Build history of the part. All positions in model axes, mm. A direction names the side the tool comes from. Coordinates: 2 decimals unless noted, no trailing zeros. Loops run counter-clockwise (first coordinate to the right, second up) from the corner with the lowest first, then second, coordinate; pieces in that order, holes last.
(1) Slice it at B-B (x = 5). Give the number of separate pieces and of enclosed holes in the cut face, and give its area (3 significant figures).
(2) Flat gauge pins, fed straight in: P1, Ø3, axis at x = 20.5, z = 56, coming from the +Y side; P2, Ø8, axis at x = 5.5, y = 6, coming from the +Z side; P3, Ø12, axis at x = 9.5, y = 16, coming from the +Z side. Where does each tip first touch, or does it go through?
(3) Slice it at C-C (z = 70). Give the cut face in (x, y).
(4) Tool access for faces 5 (the face through (25, -18, 32)), 6 (the face through (5, -45, 67)), 7 (the face through (3.7, 3.7, 3)): list every direction of +Z, -Z, +X, -X, +Y, -Y with a clear straight run to the whole face (end or side of a thin tool).
(5) Wall check: L1, parallel to X at y = 5, z = 16.25; L2, parallel to X at y = -47.6, z = 70; L3, parallel to Z at x = 20, y = -49.15. Give the ranges that are in metal, low to high.
(6) Slice it at A-A (y = 5). Give the cut face in (x, z), and give its area (3 significant figures).
(7) Two-plate mould, pull along Z, no slides. Class faces 1 (the face through (19, 18, 3)), 2 (the face through (19.792, -48.521, 71.586)), 3 (the face through (6.3, -47, 53.7)), 4 (the face through (12, 13, 0)): pulls with the +Z half, pulls with the -Z half, needs draft (parallel to the pull), parting line crosses it, or undercut.
from build123d import *

# Parameters (mm, degrees)
BOSS_EXTRUDE1_DEPTH = 25
CUT_EXTRUDE2_REACH  = 80
CUT_EXTRUDE2_START  = -3
SKETCH2_R           = 3
SKETCH2_R_2         = 1.6
CUT_EXTRUDE3_REACH  = 77
SKETCH2_3_R         = 1.6
CUT_EXTRUDE7_REACH  = 80
CUT_EXTRUDE7_START  = -3
SKETCH3_R           = 3
SKETCH3_R_2         = 1.6
CUT_EXTRUDE8_REACH  = 77
SKETCH3_3_R         = 1.6


with BuildPart() as part:
    # Sketch1 → Boss-Extrude1 (new body)
    with BuildSketch(Plane(origin=(0, 0, 0), x_dir=(0, 0, -1), z_dir=(1, 0, 0))):
        Polygon((0, 0), (-50, -50), (-75, -50), (0, 25), align=None)
    extrude(amount=BOSS_EXTRUDE1_DEPTH)

    # Sketch2 → Cut-Extrude2 (cut, up to next)
    with BuildSketch(Plane.XZ.offset(50).offset(CUT_EXTRUDE2_START), mode=Mode.PRIVATE) as cut_extrude2_sk1:
        with Locations((20, 70)):
            Circle(SKETCH2_R)
        with Locations((20, 70)):
            Circle(SKETCH2_R_2, mode=Mode.SUBTRACT)
    cut_extrude2_tool1 = extrude(cut_extrude2_sk1.sketch, amount=-CUT_EXTRUDE2_REACH, mode=Mode.PRIVATE) & part.part
    add(cut_extrude2_tool1.solids().sort_by_distance((17.084853, -47, 70))[0], mode=Mode.SUBTRACT)
    # Sketch2 → Cut-Extrude2 (cut, up to next)
    with BuildSketch(Plane.XZ.offset(50).offset(CUT_EXTRUDE2_START), mode=Mode.PRIVATE) as cut_extrude2_sk2:
        with Locations((5, 70)):
            Circle(SKETCH2_R)
        with Locations((5, 70)):
            Circle(SKETCH2_R_2, mode=Mode.SUBTRACT)
    cut_extrude2_tool2 = extrude(cut_extrude2_sk2.sketch, amount=-CUT_EXTRUDE2_REACH, mode=Mode.PRIVATE) & part.part
    add(cut_extrude2_tool2.solids().sort_by_distance((2.084853, -47, 70))[0], mode=Mode.SUBTRACT)
    # Sketch2 → Cut-Extrude2 (cut, up to next)
    with BuildSketch(Plane.XZ.offset(50).offset(CUT_EXTRUDE2_START), mode=Mode.PRIVATE) as cut_extrude2_sk3:
        with Locations((5, 55)):
            Circle(SKETCH2_R)
        with Locations((5, 55)):
            Circle(SKETCH2_R_2, mode=Mode.SUBTRACT)
    cut_extrude2_tool3 = extrude(cut_extrude2_sk3.sketch, amount=-CUT_EXTRUDE2_REACH, mode=Mode.PRIVATE) & part.part
    add(cut_extrude2_tool3.solids().sort_by_distance((2.084853, -47, 55))[0], mode=Mode.SUBTRACT)
    # Sketch2 → Cut-Extrude2 (cut, up to next)
    with BuildSketch(Plane.XZ.offset(50).offset(CUT_EXTRUDE2_START), mode=Mode.PRIVATE) as cut_extrude2_sk4:
        with Locations((20, 55)):
            Circle(SKETCH2_R)
        with Locations((20, 55)):
            Circle(SKETCH2_R_2, mode=Mode.SUBTRACT)
    cut_extrude2_tool4 = extrude(cut_extrude2_sk4.sketch, amount=-CUT_EXTRUDE2_REACH, mode=Mode.PRIVATE) & part.part
    add(cut_extrude2_tool4.solids().sort_by_distance((17.084853, -47, 55))[0], mode=Mode.SUBTRACT)

    # Sketch2_3 → Cut-Extrude3 (cut, up to next)
    with BuildSketch(Plane.XZ.offset(50), mode=Mode.PRIVATE) as cut_extrude3_sk1:
        with Locations((20, 70)):
            Circle(SKETCH2_3_R)
    cut_extrude3_tool1 = extrude(cut_extrude3_sk1.sketch, amount=-CUT_EXTRUDE3_REACH, mode=Mode.PRIVATE) & part.part
    add(cut_extrude3_tool1.solids().sort_by_distance((20, -50, 70))[0], mode=Mode.SUBTRACT)
    # Sketch2_3 → Cut-Extrude3 (cut, up to next)
    with BuildSketch(Plane.XZ.offset(50), mode=Mode.PRIVATE) as cut_extrude3_sk2:
        with Locations((5, 70)):
            Circle(SKETCH2_3_R)
    cut_extrude3_tool2 = extrude(cut_extrude3_sk2.sketch, amount=-CUT_EXTRUDE3_REACH, mode=Mode.PRIVATE) & part.part
    add(cut_extrude3_tool2.solids().sort_by_distance((5, -50, 70))[0], mode=Mode.SUBTRACT)
    # Sketch2_3 → Cut-Extrude3 (cut, up to next)
    with BuildSketch(Plane.XZ.offset(50), mode=Mode.PRIVATE) as cut_extrude3_sk3:
        with Locations((5, 55)):
            Circle(SKETCH2_3_R)
    cut_extrude3_tool3 = extrude(cut_extrude3_sk3.sketch, amount=-CUT_EXTRUDE3_REACH, mode=Mode.PRIVATE) & part.part
    add(cut_extrude3_tool3.solids().sort_by_distance((5, -50, 55))[0], mode=Mode.SUBTRACT)
    # Sketch2_3 → Cut-Extrude3 (cut, up to next)
    with BuildSketch(Plane.XZ.offset(50), mode=Mode.PRIVATE) as cut_extrude3_sk4:
        with Locations((20, 55)):
            Circle(SKETCH2_3_R)
    cut_extrude3_tool4 = extrude(cut_extrude3_sk4.sketch, amount=-CUT_EXTRUDE3_REACH, mode=Mode.PRIVATE) & part.part
    add(cut_extrude3_tool4.solids().sort_by_distance((20, -50, 55))[0], mode=Mode.SUBTRACT)

    # Sketch3 → Cut-Extrude7 (cut, up to next)
    with BuildSketch(Plane(origin=(0, 0, 0), x_dir=(-1, 0, 0), z_dir=(0, 0, -1)).offset(CUT_EXTRUDE7_START), mode=Mode.PRIVATE) as cut_extrude7_sk1:
        with Locations((-20, 20)):
            Circle(SKETCH3_R)
        with Locations((-20, 20)):
            Circle(SKETCH3_R_2, mode=Mode.SUBTRACT)
    cut_extrude7_tool1 = extrude(cut_extrude7_sk1.sketch, amount=-CUT_EXTRUDE7_REACH, mode=Mode.PRIVATE) & part.part
    add(cut_extrude7_tool1.solids().sort_by_distance((22.915147, 20, 3))[0], mode=Mode.SUBTRACT)
    # Sketch3 → Cut-Extrude7 (cut, up to next)
    with BuildSketch(Plane(origin=(0, 0, 0), x_dir=(-1, 0, 0), z_dir=(0, 0, -1)).offset(CUT_EXTRUDE7_START), mode=Mode.PRIVATE) as cut_extrude7_sk2:
        with Locations((-20, 5)):
            Circle(SKETCH3_R)
        with Locations((-20, 5)):
            Circle(SKETCH3_R_2, mode=Mode.SUBTRACT)
    cut_extrude7_tool2 = extrude(cut_extrude7_sk2.sketch, amount=-CUT_EXTRUDE7_REACH, mode=Mode.PRIVATE) & part.part
    add(cut_extrude7_tool2.solids().sort_by_distance((22.915147, 5, 3))[0], mode=Mode.SUBTRACT)
    # Sketch3 → Cut-Extrude7 (cut, up to next)
    with BuildSketch(Plane(origin=(0, 0, 0), x_dir=(-1, 0, 0), z_dir=(0, 0, -1)).offset(CUT_EXTRUDE7_START), mode=Mode.PRIVATE) as cut_extrude7_sk3:
        with Locations((-5, 5)):
            Circle(SKETCH3_R)
        with Locations((-5, 5)):
            Circle(SKETCH3_R_2, mode=Mode.SUBTRACT)
    cut_extrude7_tool3 = extrude(cut_extrude7_sk3.sketch, amount=-CUT_EXTRUDE7_REACH, mode=Mode.PRIVATE) & part.part
    add(cut_extrude7_tool3.solids().sort_by_distance((7.915147, 5, 3))[0], mode=Mode.SUBTRACT)
    # Sketch3 → Cut-Extrude7 (cut, up to next)
    with BuildSketch(Plane(origin=(0, 0, 0), x_dir=(-1, 0, 0), z_dir=(0, 0, -1)).offset(CUT_EXTRUDE7_START), mode=Mode.PRIVATE) as cut_extrude7_sk4:
        with Locations((-5, 20)):
            Circle(SKETCH3_R)
        with Locations((-5, 20)):
            Circle(SKETCH3_R_2, mode=Mode.SUBTRACT)
    cut_extrude7_tool4 = extrude(cut_extrude7_sk4.sketch, amount=-CUT_EXTRUDE7_REACH, mode=Mode.PRIVATE) & part.part
    add(cut_extrude7_tool4.solids().sort_by_distance((7.915147, 20, 3))[0], mode=Mode.SUBTRACT)

    # Sketch3_3 → Cut-Extrude8 (cut, up to next)
    with BuildSketch(Plane(origin=(0, 0, 0), x_dir=(-1, 0, 0), z_dir=(0, 0, -1)), mode=Mode.PRIVATE) as cut_extrude8_sk1:
        with Locations((-20, 20)):
            Circle(SKETCH3_3_R)
    cut_extrude8_tool1 = extrude(cut_extrude8_sk1.sketch, amount=-CUT_EXTRUDE8_REACH, mode=Mode.PRIVATE) & part.part
    add(cut_extrude8_tool1.solids().sort_by_distance((20, 20, 0))[0], mode=Mode.SUBTRACT)
    # Sketch3_3 → Cut-Extrude8 (cut, up to next)
    with BuildSketch(Plane(origin=(0, 0, 0), x_dir=(-1, 0, 0), z_dir=(0, 0, -1)), mode=Mode.PRIVATE) as cut_extrude8_sk2:
        with Locations((-20, 5)):
            Circle(SKETCH3_3_R)
    cut_extrude8_tool2 = extrude(cut_extrude8_sk2.sketch, amount=-CUT_EXTRUDE8_REACH, mode=Mode.PRIVATE) & part.part
    add(cut_extrude8_tool2.solids().sort_by_distance((20, 5, 0))[0], mode=Mode.SUBTRACT)
    # Sketch3_3 → Cut-Extrude8 (cut, up to next)
    with BuildSketch(Plane(origin=(0, 0, 0), x_dir=(-1, 0, 0), z_dir=(0, 0, -1)), mode=Mode.PRIVATE) as cut_extrude8_sk3:
        with Locations((-5, 5)):
            Circle(SKETCH3_3_R)
    cut_extrude8_tool3 = extrude(cut_extrude8_sk3.sketch, amount=-CUT_EXTRUDE8_REACH, mode=Mode.PRIVATE) & part.part
    add(cut_extrude8_tool3.solids().sort_by_distance((5, 5, 0))[0], mode=Mode.SUBTRACT)
    # Sketch3_3 → Cut-Extrude8 (cut, up to next)
    with BuildSketch(Plane(origin=(0, 0, 0), x_dir=(-1, 0, 0), z_dir=(0, 0, -1)), mode=Mode.PRIVATE) as cut_extrude8_sk4:
        with Locations((-5, 20)):
            Circle(SKETCH3_3_R)
    cut_extrude8_tool4 = extrude(cut_extrude8_sk4.sketch, amount=-CUT_EXTRUDE8_REACH, mode=Mode.PRIVATE) & part.part
    add(cut_extrude8_tool4.solids().sort_by_distance((5, 20, 0))[0], mode=Mode.SUBTRACT)


solid = part.part
Response values:
1. separate pieces: 5
1. enclosed holes: 0
1. area: 1,300 mm2
2. P1: stops at y = -47
2. P2: stops at z = 23
2. P3: stops at z = 15
3. outline: (0, -50) - (3.4, -50) - (3.4, -47) - (2, -47) - (2, -45) - (0, -45) - close; (6.6, -50) - (18.4, -50) - (18.4, -47) - (17, -47) - (17, -45) - (8, -45) - (8, -47) - (6.6, -47) - close; (21.6, -50) - (25, -50) - (25, -45) - (23, -45) - (23, -47) - (21.6, -47) - close
4. face 5: +Z, -Z, +X, +Y, -Y
4. face 6: +Y
4. face 7: +Z
5. L1: x = 0 to 2, 8 to 17, 23 to 25
5. L2: x = 0 to 3.4, 6.6 to 18.4, 21.6 to 25
5. L3: z = 49.15 to 53.4, 56.6 to 68.4, 71.6 to 74.15
6. outline: (0, 0) - (3.4, 0) - (3.4, 3) - (2, 3) - (2, 20) - (0, 20) - close; (6.6, 0) - (18.4, 0) - (18.4, 3) - (17, 3) - (17, 20) - (8, 20) - (8, 3) - (6.6, 3) - close; (21.6, 0) - (25, 0) - (25, 20) - (23, 20) - (23, 3) - (21.6, 3) - close
6. area: 277 mm2
7. face 1: pulls with the +Z half
7. face 2: undercut
7. face 3: undercut
7. face 4: pulls with the -Z half
